Autodesk Inventor part; units mm, degrees
ref_plane "YZ Plane" through (0, 0, 0) normal (1, 0, 0) x (0, 1, 0)
ref_plane "XZ Plane" through (0, 0, 0) normal (0, 1, 0) x (-1, 0, 0)
ref_plane "XY Plane" through (0, 0, 0) normal (0, 0, 1) x (1, 0, 0)
sketch "Эскиз1" plane through (0, 0, 0) normal (1, 0, 0) x (0, 1, 0)
  line L0 (0, 0) -> (0, 31)
  line L1 (0, 0) -> (0, -31)
  circle A0 centre (0, 31) radius 2
  circle A1 centre (0, -31) radius 2
  line L2 (-5, 35) -> (5, 35)
  line L3 (5, 35) -> (5, -35)
  line L4 (5, -35) -> (-5, -35)
  line L5 (-5, -35) -> (-5, 35)
  line L6 (-5, 35) -> (5, -35) construction
  line L7 (5, 35) -> (-5, -35) construction
  dimension "d0" = 31
  dimension "d1" = 31
  dimension "d2" = 4
  dimension "d3" = 4
  dimension "d4" = 10
  dimension "d5" = 70
extrude "Выдавливание1" add sketch "Эскиз1" along normal blind 3
sketch "Эскиз2" plane through (3, 0, 0) normal (1, 0, 0) x (0, 0, -1)
  line L0 (35, 5) -> (-35, 5)
  line L1 (0, 5) -> (-14, 5)
  line L2 (-14, 5) -> (14, 5)
  line L3 (-14, 5) -> (-14, 10.5)
  line L4 (-14, 5) -> (-19, 5)
  line L5 (-19, 5) -> (19, 5)
  line L6 (19, 5) -> (19, 55)
  line L7 (19, 55) -> (-19, 55)
  line L8 (-19, 55) -> (-19, 5)
  circle A0 centre (-14, 10.5) radius 2
  line L9 (19, 30) -> (-19, 30)
  line L10 (0, 30) -> (0, 26.3042)
  circle A1 centre (14, 10.5) radius 2
  circle A2 centre (-14, 49.5) radius 2
  circle A3 centre (14, 49.5) radius 2
  point P0 (0, 0)
  dimension "d8" = 14
  dimension "d9" = 28
  dimension "d10" = 5.5
  dimension "d11" = 5
  dimension "d12" = 38
  dimension "d13" = 50
  dimension "d14" = 4
extrude "Выдавливание2" add sketch "Эскиз2" against normal blind 3
equation "\"d1\" = d0"
properties part number "КВ33.044.704 - Панель установки принимающей платы оси Y"
The listing builds one solid part. Answer for the finished solid, in the listing's coordinates (mm). A direction names the side the tool comes from. Coordinates: 2 decimals unless noted, no trailing zeros. Write each loop counter-clockwise with the first axis right and the second up, starting at its lowest first coordinate (ties: lowest second). Pieces come first, ordered by that corner, then holes. Notation, with made-up numbers: (3.5, -10) - (48.5, -10) arc R17 cw to (48.5, 0) - close; hole circle Ø2 at (15, -10). An arc over 180 degrees is marked (long way). Return JSON: item names as keys, results as strings. Group by question number.
Q1. The part is cut by section B-B on y = 0. Write down the section's boundary in (x, z).
Q2. The part is cut by section D-D on x = 0.65. Write down the section's boundary in (y, z).
Q3. The part is cut by section A-A on z = 31. Write down the section's boundary in (x, y).
Q4. Which of the six approach directions +Z, -Z, +X, -X, +Y, -Y give full straight-line access (tool end or side, diameter ignored) to faces 1 (the flat face through (2, 30, 19)), 2 (the cylindrical face through (1.521, 12.483, -13.74)), 3 (the flat face through (1, 5, -27))?
Q5. Find the intervals of material crossed by line 1 along Y through (x, z) = (1.35, -14); line 2 along Z through (x, y) = (1.65, 0); line 3 along Y through (x, z) = (1.95, 31), in increasing order. Write a range as [from, to].
Q6. A flat-ended cylindrical pin translates along its axis: pin 1 Ø0.9 at (x, y) = (1, 21) entering from -Z. Find the tip coordinate at first contact, or state that the pin passes through.
Q7. The part is cut by section C-C on z = 14. Write down the section's boundary in (x, y), and give its area (3 significant figures).
Q8. For a pull along Z with two mould halves and no side action, classify faces 4 (the flat face through (2, 30, -19)), 5 (the cylindrical face through (1, 0, 33)), 6 (the flat face through (1, 5, 27)) as +Z half, -Z half, draft (parallel to the pull), parting line (faces both ways), or undercut.
Evaluation:
{
 "1": {"outline": "(0, -35) - (3, -35) - (3, -33) - (0, -33) - close; (0, -29) - (3, -29) - (3, 29) - (0, 29) - close; (0, 33) - (3, 33) - (3, 35) - (0, 35) - close"},
 "2": {"outline": "(-5, -35) - (5, -35) - (5, -19) - (55, -19) - (55, 19) - (5, 19) - (5, 35) - (-5, 35) - close; hole circle Ø4 at (0, -31); hole circle Ø4 at (0, 31); hole circle Ø4 at (10.5, -14); hole circle Ø4 at (10.5, 14); hole circle Ø4 at (49.5, -14); hole circle Ø4 at (49.5, 14)"},
 "3": {"outline": "(0, -5) - (3, -5) - (3, -2) - (0, -2) - close; (0, 2) - (3, 2) - (3, 5) - (0, 5) - close"},
 "4": {"face 1": "+Z, +X, -X, +Y", "face 2": "+X, -X", "face 3": "-Z, +X, -X, +Y"},
 "5": {"line 1": "y = [-5, 8.5], [12.5, 47.5], [51.5, 55]", "line 2": "z = [-35, -33], [-29, 29], [33, 35]", "line 3": "y = [-5, -2], [2, 5]"},
 "6": {"pin 1": "stops at z = -19"},
 "7": {"outline": "(0, -5) - (3, -5) - (3, 8.5) - (0, 8.5) - close; (0, 12.5) - (3, 12.5) - (3, 47.5) - (0, 47.5) - close; (0, 51.5) - (3, 51.5) - (3, 55) - (0, 55) - close", "area": "156 mm2"},
 "8": {"face 4": "-Z half", "face 5": "undercut", "face 6": "draft"}
}
